from build123d import *

# Parameters (mm, degrees)
F0_W     = 50
F0_H     = 3
F1_DEPTH = 10
F3_DEPTH = 55.5734787771
F4_W     = 3
F4_H     = 0.4
F5_REACH = 58.6000279672


with BuildPart() as f1:
    # F0 (on Top) → F1 (new body)
    with BuildSketch(Plane.XY):
        Rectangle(F0_W, F0_H)
    extrude(amount=F1_DEPTH)


with BuildPart() as f1b:
    # F0 (on Top) → F1, piece 2 (new body)
    with BuildSketch(Plane.XY):
        Polygon((-26.5434872663, 24.0724787771), (-25, 21.5), (25, 51.5), (23.4565127337, 54.0724787771), align=None)
    extrude(amount=F1_DEPTH)


with BuildPart() as f3_tool:
    # F2 (on face) → F3 (new body, through all)
    with BuildSketch(Plane.XZ.offset(1.5)):
        Polygon((17.6366446762, 10), (-26.5434872663, 10), (-26.5434872663, 1.4285714286), (-19.1801319425, 1.4285714286), (-19.1801319425, 2.8571428571), (-11.8167766188, 2.8571428571), (-11.8167766188, 4.2857142857), (-4.453421295, 4.2857142857), (-4.453421295, 5.7142857143), (2.9099340287, 5.7142857143), (2.9099340287, 7.1428571429), (10.2732893525, 7.1428571429), (10.2732893525, 8.5714285714), (17.6366446762, 8.5714285714), align=None)
    extrude(amount=-F3_DEPTH)


with BuildPart() as f1_1:
    add(f1.part)

    # F3: cut by f3_tool
    add(f3_tool.part, mode=Mode.SUBTRACT)



with BuildPart() as f1b_1:
    add(f1b.part)

    # F3: cut by f3_tool
    add(f3_tool.part, mode=Mode.SUBTRACT)


with BuildPart() as f1_2:
    add(f1_1.part)

    add(f1b_1.part)  # F5 merges F1b
    f5_end = f1_2.faces().sort_by_distance((5.616262324, 43.3683285313, 3.4924250952))[0]
    # F4 (on face) → F5 (join, up to a face of the model that its end follows)
    with BuildSketch(Plane.XZ.offset(1.5)):
        with Locations((-22.0900659713, 1.2285714286)):
            Rectangle(F4_W, F4_H)
        with Locations((-15.4984542807, 2.6571428571)):
            Rectangle(F4_W, F4_H)
        with Locations((-8.1350989569, 4.0857142857)):
            Rectangle(F4_W, F4_H)
        with Locations((-0.7717436331, 5.5142857143)):
            Rectangle(F4_W, F4_H)
        with Locations((6.5916116906, 6.9428571429)):
            Rectangle(F4_W, F4_H)
        with Locations((13.9549670144, 8.3714285714)):
            Rectangle(F4_W, F4_H)
        with Locations((21.3183223381, 9.8)):
            Rectangle(F4_W, F4_H)
    f5_long = extrude(amount=-F5_REACH, mode=Mode.PRIVATE)
    add(split(f5_long, bisect_by=f5_end, keep=Keep.BOTTOM, mode=Mode.PRIVATE))


solid = f1_2.part
Geometry check sheet. Reference: the model listing, model coordinates, mm. A direction names the side the tool comes from. Round coordinates to 2 decimals unless told otherwise and drop trailing zeros. Order: outer loops, then holes, each group sorted by start corner. A loop starts at its lowest first (then second) coordinate and runs counter-clockwise, first axis right, second up. Notation, with made-up numbers: M 60.25,47.25 L 98.25,47.25 A30 cw 98.25,85.25 Z; hole C -31.75,28 d11. An arc over 180 degrees is marked long. Answer in a Markdown table with one row per item.
(1) Draft check along Y on faces 1 (the face through (10.273, 0, 8)), 2 (the face through (4.362, 42.616, 3.819)), 3 (the face through (-16, 15, 2.457)), 4 (the face through (-22, 13, 1.029)). Enter one of: released by +Y, released by -Y, zero draft, split by the parting line, or undercut.
Responses:
| item | result |
|---|---|
| face 1 | zero draft |
| face 2 | released by +Y |
| face 3 | undercut |
| face 4 | undercut |
(2) Sectioned sample at A-A, the plane y = 15.5. Record the cut outline in (x, z).
Responses:
| item | result |
|---|---|
| outline | M -23.59,1.03 L -20.59,1.03 L -20.59,1.43 L -23.59,1.43 Z; M -17,2.46 L -14,2.46 L -14,2.86 L -17,2.86 Z; M -9.64,3.89 L -6.64,3.89 L -6.64,4.29 L -9.64,4.29 Z; M -2.27,5.31 L 0.73,5.31 L 0.73,5.71 L -2.27,5.71 Z; M 5.09,6.74 L 8.09,6.74 L 8.09,7.14 L 5.09,7.14 Z; M 12.45,8.17 L 15.45,8.17 L 15.45,8.57 L 12.45,8.57 Z; M 19.82,9.6 L 22.82,9.6 L 22.82,10 L 19.82,10 Z |
(3) Sectioned sample at B-B, the plane x = -22.5. Record the cut outline in (y, z).
Responses:
| item | result |
|---|---|
| outline | M -1.5,0 L 1.5,0 L 1.5,1.03 L 23,1.03 L 23,0 L 26.5,0 L 26.5,1.43 L -1.5,1.43 Z |
(4) Tool access check on faces 5 (the face through (0, 0, 0)), 6 (the face through (-19.18, 27, 2)), 7 (the face through (-25, 0, 1)). Record the directions out of +Z, -Z, +X, -X, +Y, -Y that give a thin tool (end or side, any length) a straight path to the whole face; none if there is none.
Responses:
| item | result |
|---|---|
| face 5 | -Z, +X, -X, +Y, -Y |
| face 6 | +Z, -X, +Y, -Y |
| face 7 | +Z, -Z, -X, -Y |
(5) Sectioned sample at C-C, the plane x = 21.5. Record the cut outline in (y, z), and give its area (3 significant figures).
Responses:
| item | result |
|---|---|
| outline | M -1.5,0 L 1.5,0 L 1.5,9.6 L 49.4,9.6 L 49.4,0 L 52.9,0 L 52.9,10 L -1.5,10 Z |
| area | 84.1 mm² |
(6) Go/stop test with flat-tipped pins: P1, Ø6, axis at x = -1, y = 22.5, coming from the +Z side; P2, Ø3.5, axis at x = 5, y = 32, coming from the +Z side; P3, Ø1.5, axis at y = 42, z = 4.5, coming from the +X side. Record where each tip stops, or that it passes through.
Responses:
| item | result |
|---|---|
| P1 | stops at z = 5.71 |
| P2 | stops at z = 7.14 |
| P3 | stops at x = 10.42 |
(7) Scan lines: probe 1 along Z at (x, y) = (22, 15); probe 2 along X at (y, z) = (1, 9.25); probe 3 along Y at (x, z) = (19.5, 4.75). Record each from-to range of solid material in increasing order. Write a range as from..to.
Responses:
| item | result |
|---|---|
| probe 1 | z = 9.6..10 |
| probe 2 | x = 17.64..25 |
| probe 3 | y = -1.5..1.5, 48.2..51.7 |
